from build123d import *

# Parameters (mm, degrees)
F0_R     = 0.7
F1_DEPTH = 2
F2_R     = 1
F2_R_2   = 0.7
F3_DEPTH = 1.5
F4_R     = 1.5
F4_R_2   = 1
F5_DEPTH = 36.75
F6_R     = 1
F7_DEPTH = 1.5
F8_R     = 0.7
F9_DEPTH = 2
F10_SIZE = 0.2
F11_SIZE = 0.1


with BuildPart() as f1:
    # F0 (on Top) → F1 (new body)
    with BuildSketch(Plane.XY):
        Circle(F0_R)
    extrude(amount=F1_DEPTH)

    # F2 (on face) → F3 (join)
    with BuildSketch(Plane.XY.offset(2)):
        Circle(F2_R)
        Circle(F2_R_2, mode=Mode.SUBTRACT)
        Circle(F2_R_2)
    extrude(amount=F3_DEPTH)

    # F4 (on face) → F5 (join)
    with BuildSketch(Plane.XY.offset(3.5)):
        Circle(F4_R)
        Circle(F4_R_2, mode=Mode.SUBTRACT)
        Circle(F4_R_2)
    extrude(amount=F5_DEPTH)

    # F6 (on face) → F7 (join)
    with BuildSketch(Plane.XY.offset(40.25)):
        Circle(F6_R)
    extrude(amount=F7_DEPTH)

    # F8 (on face) → F9 (join)
    with BuildSketch(Plane.XY.offset(41.75)):
        Circle(F8_R)
    extrude(amount=F9_DEPTH)

    # F10
    f10_edges = [f1.edges().sort_by_distance(p)[0] for p in [
        (-0.7, 0, 0),
        (-0.7, 0, 43.75),
    ]]
    chamfer(f10_edges, length=F10_SIZE)

    # F11
    f11_edges = [f1.edges().sort_by_distance(p)[0] for p in [
        (-1.5, 0, 40.25),
        (-1.5, 0, 3.5),
    ]]
    chamfer(f11_edges, length=F11_SIZE)


solid = f1.part
Verification items for the finished model (mm, model axes). A direction names the side the tool comes from. Give positions to 0.01 mm unless a question says otherwise; leave off trailing zeros. Order: outer loops, then holes, each group sorted by start corner. A loop starts at its lowest first (then second) coordinate and runs counter-clockwise, first axis right, second up. Notation, with made-up numbers: M -10.75,-2.5 L 44.25,-2.5 A29 cw 44.25,23.5 Z; hole C 63.5,22.25 d10. An arc over 180 degrees is marked long. Use one line per item in the form item = value. Start each with the question number.
Q1. Access from +Z, -Z, +X, -X, +Y, -Y to the whole of each face (thin tool, end or side, straight path). Record for faces 1 (the cylindrical face through (0, -1, 41)), 2 (the flat face through (0, 0, 0)), 3 (the cylindrical face through (0, -1, 3)).
Q2. Section check A-A (y = 0). Enter the section's corners in (x, z), then the cut area to 3 significant figures.
Q3. Scan lines: line 1 along Z through (x, y) = (0.4, 1.25); line 2 along Z through (x, y) = (0.2, -0.9); line 3 along Y through (x, z) = (0.15, 12.5). Record each from-to range of solid material in increasing order. Write a range as [from, to].
Q4. Section check C-C (z = 10.5). Enter the section's corners in (x, y).
Q5. Go/stop test with flat-tipped pins: pin 1 Ø1 at (x, z) = (-1, 32) entering from +Y; pin 2 Ø1 at (x, y) = (0.5, -1) entering from +Z. Record where each tip stops, or that it passes through.
Evaluation:
q1.face_1 = +Z
q1.face_2 = -Z, +X, -X, +Y, -Y
q1.face_3 = -Z
q2.outline = M -1.5,3.6 L -1.4,3.5 L -1,3.5 L -1,2 L -0.7,2 L -0.7,0.2 L -0.5,0 L 0.5,0 L 0.7,0.2 L 0.7,2 L 1,2 L 1,3.5 L 1.4,3.5 L 1.5,3.6 L 1.5,40.15 L 1.4,40.25 L 1,40.25 L 1,41.75 L 0.7,41.75 L 0.7,43.55 L 0.5,43.75 L -0.5,43.75 L -0.7,43.55 L -0.7,41.75 L -1,41.75 L -1,40.25 L -1.4,40.25 L -1.5,40.15 Z
q2.area = 122 mm2
q3.line_1 = [3.5, 40.25]
q3.line_2 = [2, 41.75]
q3.line_3 = [-1.49, 1.49]
q4.outline = C 0,0 d3
q5.pin_1 = 1.41
q5.pin_2 = 43.63
